from build123d import *

# Parameters (mm, degrees)
F1_START = -55
F1_DEPTH = 415
F2_SIZE2 = 14.5
F2_SIZE  = 14.5


with BuildPart() as f1:
    # F0 (on Front) → F1 (new body)
    with BuildSketch(Plane.XZ.offset(F1_START)):
        Polygon((-4.6, -740), (-4.6, -827), (24.6, -827), (24.6, -740), (24.6, -725), (24.6, -365), (24.6, -350), (24.6, 10), (24.6, 25), (24.6, 385), (-4.6, 385), (-4.6, 25), (-4.6, 10), (-4.6, -350), (-4.6, -365), (-4.6, -725), align=None)
    extrude(amount=-F1_DEPTH)

    # F2
    f2_edges = [f1.edges().sort_by_distance(p)[0] for p in [
        (-4.6, 55, -221),
        (10, 55, -827),
        (24.6, 55, -221),
        (10, 55, 385),
    ]]
    chamfer(f2_edges, length=F2_SIZE, length2=F2_SIZE2)


solid = f1.part
Build history of the part. All positions in model axes, mm. Coordinates: 2 decimals unless noted, no trailing zeros. Order: outer loops, then holes, each group sorted by start corner. A loop starts at its lowest first (then second) coordinate and runs counter-clockwise, first axis right, second up. Notation, with made-up numbers: (40, -7.75) - (50, -7.75) arc R13 cw to (50, -0.75) - close; hole circle Ø11 at (-38, -22). An arc over 180 degrees is marked (long way). Put each result on its own line as item: value.
1. Saw through at B-B (x = 1). Write the cut outline in (y, z).
Answer sheet:
outline: (63.9, -821.4) - (69.5, -827) - (470, -827) - (470, 385) - (69.5, 385) - (63.9, 379.4) - close
2. Saw through at A-A (z = 219.5). Write the cut outline in (x, y), and give its area (3 significant figures).
Answer sheet:
outline: (-4.6, 69.5) - (9.9, 55) - (10.1, 55) - (24.6, 69.5) - (24.6, 470) - (-4.6, 470) - close
area: 11,900 mm^2
3. Drop a flat-ended pin along its axis: P1, Ø1.5, axis at x = 18.5, z = -465.5, coming from the -Y side. Give the stop position or say it passes through.
Answer sheet:
P1: stops at y = 62.65
4. Probe line 1 along Y through (x, z) = (19, 62); line 2 along Y through (x, z) = (21.25, -516). List the from-to ranges inside material, lowest first. Write a range as [from, to].
Answer sheet:
line 1: y = [63.9, 470]
line 2: y = [66.15, 470]
